Geometry check sheet. Reference: the model listing, model coordinates, mm. Face numbers are marked on the shaded views. A direction names the side the tool comes from. Round coordinates to 2 decimals unless told otherwise and drop trailing zeros. Order: outer loops, then holes, each group sorted by start corner. A loop starts at its lowest first (then second) coordinate and runs counter-clockwise, first axis right, second up. Notation, with made-up numbers: (-10, -23) - (38, -23) arc R4 ccw to (38, -17) - close; hole circle Ø4 at (59.25, -32). An arc over 180 degrees is marked (long way). Return JSON: item names as keys, results as strings. Group by question number.
Q1. Sectioned sample at B-B, the plane y = 28. Record the cut outline in (x, z), then the cut area to 3 significant figures.
Q2. Draft check along X on the marked faces 4, 5 and 6. Enter one of: pulls with the +X half, pulls with the -X half, needs draft (parallel to the pull), parting line crosses it, or undercut.
Q3. Sectioned sample at C-C, the plane x = 0. Record the cut outline in (y, z).
Q4. Tool access check on the marked faces 1, 2 and 3. Record the directions out of +Z, -Z, +X, -X, +Y, -Y that give a thin tool (end or side, any length) a straight path to the whole face; none if there is none.
Q5. Sectioned sample at D-D, the plane y = 11. Record the cut outline in (x, z), then the cut area to 3 significant figures.
Q6. Gauge pin test, flat ends, axial feed: pin 1 Ø10 at (x, z) = (42.5, -2.5) entering from +Y; pin 2 Ø13 at (y, z) = (16, 1.5) entering from -X; pin 3 Ø10 at (y, z) = (25, 6.5) entering from +X. Record the tip position at first contact, or that the pin passes through.
Q7. Material ranges on line 1 along Z through (x, y) = (0, 41.25); line 2 along X through (y, z) = (34, -5); line 3 along Y through (x, z) = (-35.5, -7.5), recorded low to high.
Q8. Sectioned sample at A-A, the plane x = -39. Record the cut outline in (y, z).
```python
from build123d import *

# Parameters (mm, degrees)
BOSS_EXTRUDE1_DEPTH = 23
SKETCH2_R           = 17
CUT_EXTRUDE1_DEPTH  = 66.030761952
SKETCH3_R           = 6
CUT_EXTRUDE2_DEPTH  = 66.030761987
CUT_EXTRUDE3_START  = -12
CUT_EXTRUDE3_DEPTH  = 12


# Read off the part's stored shape, not the designer's step: Cut-Extrude3
with BuildPart() as part:
    # Sketch1 → Boss-Extrude1 (new, symmetric)
    with BuildSketch(Plane.XY):
        with BuildLine():
            Line((-32.062618722, 8), (-22.627416998, 8))
            ThreePointArc((-22.627416998, 8), (0, 24), (22.627416998, 8))
            Line((22.627416998, 8), (32.062618722, 8))
            Line((32.062618722, 8), (32.062618722, 24))
            Line((32.062618722, 24), (54, 24))
            Line((54, 24), (54, 36))
            Line((54, 36), (32.391338275, 36))
            ThreePointArc((32.391338275, 36), (0, 48.427252609), (-32.391338275, 36))
            Line((-32.391338275, 36), (-54, 36))
            Line((-54, 36), (-54, 24))
            Line((-54, 24), (-32.062618722, 24))
            Line((-32.062618722, 24), (-32.062618722, 8))
        make_face()
    extrude(amount=BOSS_EXTRUDE1_DEPTH, both=True)

    # Sketch2 → Cut-Extrude1 (cut, through all)
    with BuildSketch(Plane(origin=(0, 36, 0), x_dir=(1, 0, 0), z_dir=(0, 1, 0))):
        with Locations((-39, 0)):
            Circle(SKETCH2_R)
        with Locations((39, 0)):
            Circle(SKETCH2_R)
    extrude(amount=CUT_EXTRUDE1_DEPTH, mode=Mode.SUBTRACT)

    # Sketch3 → Cut-Extrude2 (cut, through all)
    with BuildSketch(Plane(origin=(0, 36, 0), x_dir=(1, 0, 0), z_dir=(0, 1, 0))):
        with Locations(Location((-39, 0, 0), (0, 0, 270))):
            Circle(SKETCH3_R)
        with Locations(Location((39, 0, 0), (0, 0, 270))):
            Circle(SKETCH3_R)
    extrude(amount=-CUT_EXTRUDE2_DEPTH, mode=Mode.SUBTRACT)

    # Sketch4 → Cut-Revolve1 (revolve, cut)
    with BuildSketch(Plane.XY, mode=Mode.PRIVATE) as cut_revolve1_sk:
        Polygon((0, 50), (4, 50), (4, 33), (3, 33), (3, 20), (0, 20), align=None)
    revolve(cut_revolve1_sk.sketch.rotate(Axis((0, 50, 0), (0, -1, 0)), 180), axis=Axis((0, 50, 0), (0, -1, 0)), mode=Mode.SUBTRACT)

    # Cut-Extrude3 outline → Cut-Extrude3 (cut)
    with BuildSketch(Plane(origin=(0, 36, 0), x_dir=(1, 0, 0), z_dir=(0, 1, 0)).offset(CUT_EXTRUDE3_START)):
        with BuildLine():
            ThreePointArc((-54, 0), (-52.698550436, 11.784005345), (-48.856934001, 23))
            Line((-48.856934001, 23), (-54, 23))
            Line((-54, 23), (-54, 0))
        make_face()
        with BuildLine():
            ThreePointArc((-48.856934001, -23), (-52.698550436, -11.784005345), (-54, 0))
            Line((-54, 0), (-54, -23))
            Line((-54, -23), (-48.856934001, -23))
        make_face()
        with BuildLine():
            Line((54, 23), (48.856934001, 23))
            ThreePointArc((48.856934001, 23), (52.698550436, 11.784005345), (54, 0))
            Line((54, 0), (54, 23))
        make_face()
        with BuildLine():
            Line((54, -23), (54, 0))
            ThreePointArc((54, 0), (52.698550436, -11.784005345), (48.856934001, -23))
            Line((48.856934001, -23), (54, -23))
        make_face()
    extrude(amount=CUT_EXTRUDE3_DEPTH, mode=Mode.SUBTRACT)


solid = part.part
```
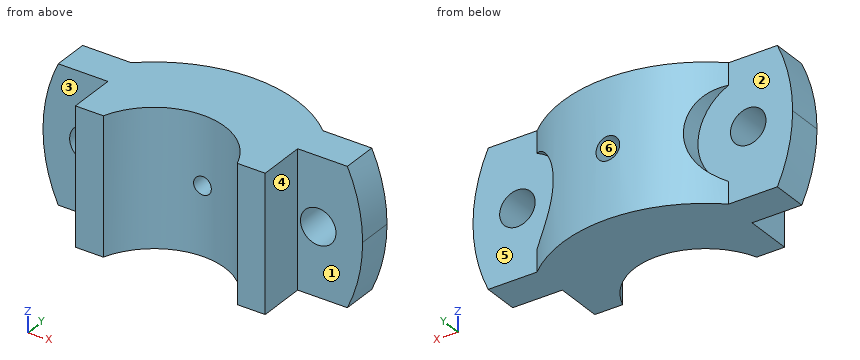
Reply:
{
 "1": {"outline": "(-48.86, -23) - (48.86, -23) arc R54 ccw to (48.86, 23) - (-48.86, 23) arc R54 ccw to start; hole circle Ø12 at (-39, 0); hole circle Ø6 at (0, 0); hole circle Ø12 at (39, 0)", "area": "4,560 mm^2"},
 "2": {"face 4": "pulls with the +X half", "face 5": "needs draft", "face 6": "undercut"},
 "3": {"outline": "(24, -23) - (48.43, -23) - (48.43, -4) - (33, -4) - (33, -3) - (24, -3) - close; (24, 3) - (33, 3) - (33, 4) - (48.43, 4) - (48.43, 23) - (24, 23) - close"},
 "4": {"face 1": "+Z, -Z, +X, -Y", "face 2": "-X, +Y", "face 3": "+Z, -Z, -X, -Y"},
 "5": {"outline": "(-32.06, -23) - (-21.33, -23) - (-21.33, 23) - (-32.06, 23) - close; (21.33, -23) - (32.06, -23) - (32.06, 23) - (21.33, 23) - close", "area": "987 mm^2"},
 "6": {"pin 1": "y = 36", "pin 2": "x = -32.06", "pin 3": "x = 53.98"},
 "7": {"line 1": "-23 to -4, 4 to 23", "line 2": "-53.77 to -42.32, -35.68 to 35.68, 42.32 to 53.77", "line 3": "24 to 36"},
 "8": {"outline": "(24, -23) - (36, -23) - (36, -6) - (24, -6) - close; (24, 6) - (36, 6) - (36, 23) - (24, 23) - close"}
}
